The listing builds one solid part. Answer for the finished solid, in the listing's coordinates (mm). Face numbers are marked on the shaded views. Coordinates: 2 decimals unless noted, no trailing zeros. Order: outer loops, then holes, each group sorted by start corner. A loop starts at its lowest first (then second) coordinate and runs counter-clockwise, first axis right, second up. Notation, with made-up numbers: (65, -3.5) -> (100, -3.5) arc R17 cw to (100, 16.5) -> close; hole circle Ø3 at (-5.5, 78.5). An arc over 180 degrees is marked (long way). Answer in a Markdown table with one row per item.
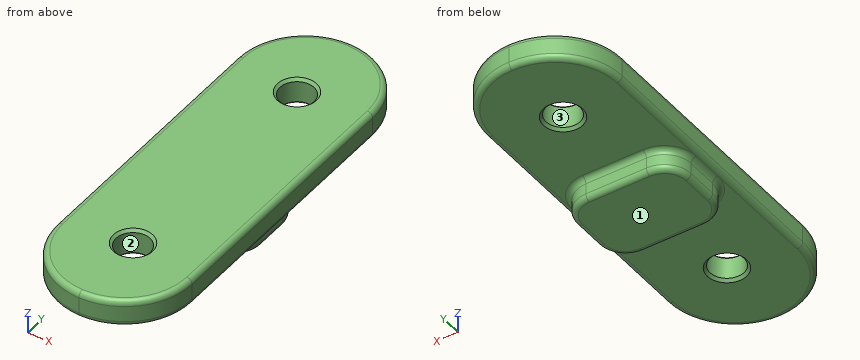
```python
from build123d import *

# Parameters (mm, degrees)
SKETCH1_W        = 25.4
SKETCH1_H        = 75.4
SKETCH1_R        = 3.2
MAINBODY_DEPTH   = 5
SKETCH2_W        = 21.4
SKETCH2_H        = 16
RIBSUPPORT_DEPTH = 4
FILLET_12_7_R    = 12.7
FILLET_5_0_R     = 5
CHAMFER_0_5_SIZE = 0.5
FILLET_1_0_R     = 1


with BuildPart() as part:
    # Sketch1 → mainBody (new body)
    with BuildSketch(Plane.XY):
        with Locations((0, 22.7)):
            Rectangle(SKETCH1_W, SKETCH1_H)
        Circle(SKETCH1_R, mode=Mode.SUBTRACT)
        with Locations((0, 45.4)):
            Circle(SKETCH1_R, mode=Mode.SUBTRACT)
    extrude(amount=MAINBODY_DEPTH)

    # Sketch2 → ribSupport (add)
    with BuildSketch(Plane(origin=(0, 0, 0), x_dir=(-1, 0, 0), z_dir=(0, 0, -1))):
        with Locations((0, 22.7)):
            Rectangle(SKETCH2_W, SKETCH2_H)
    extrude(amount=RIBSUPPORT_DEPTH)

    # Fillet-12.7
    fillet_12_7_edges = [part.edges().sort_by_distance(p)[0] for p in [
        (-12.7, -15, 2.5),
        (12.7, -15, 2.5),
        (-12.7, 60.4, 2.5),
        (12.7, 60.4, 2.5),
    ]]
    fillet(fillet_12_7_edges, radius=FILLET_12_7_R - 0.0001)  # a hair under: the kernel refuses the full size

    # Fillet-5.0
    fillet_5_0_edges = [part.edges().sort_by_distance(p)[0] for p in [
        (10.7, 30.7, -2),
        (10.7, 14.7, -2),
        (-10.7, 14.7, -2),
        (-10.7, 30.7, -2),
    ]]
    fillet(fillet_5_0_edges, radius=FILLET_5_0_R)

    # Chamfer-0.5
    chamfer_0_5_edges = [part.edges().sort_by_distance(p)[0] for p in [
        (-3.2, 0, 0),
        (-3.2, 0, 5),
        (-3.2, 45.4, 0),
        (-3.2, 45.4, 5),
    ]]
    chamfer(chamfer_0_5_edges, length=CHAMFER_0_5_SIZE)

    # Fillet-1.0
    fillet_1_0_edges = [part.edges().sort_by_distance(p)[0] for p in [
        (-12.7, 22.7, 0),
        (12.7, 22.7, 0),
        (8.98028541, 56.68028541, 0),
        (-8.98028541, 56.68028541, 0),
        (8.98028541, -11.28028541, 0),
        (-8.98028541, -11.28028541, 0),
        (-12.7, 22.7, 5),
        (12.7, 22.7, 5),
        (8.98028541, 56.68028541, 5),
        (-8.98028541, 56.68028541, 5),
        (8.98028541, -11.28028541, 5),
        (-8.98028541, -11.28028541, 5),
        (0, 30.7, 0),
        (0, 30.7, -4),
        (-10.7, 22.7, 0),
        (-10.7, 22.7, -4),
        (10.7, 22.7, -4),
        (0, 14.7, -4),
        (9.235533906, 29.235533906, -4),
        (9.235533906, 16.164466094, -4),
        (-9.235533906, 16.164466094, -4),
        (-9.235533906, 29.235533906, -4),
        (0, 14.7, 0),
        (10.7, 22.7, 0),
        (-9.235533906, 29.235533906, 0),
        (-9.235533906, 16.164466094, 0),
        (9.235533906, 16.164466094, 0),
        (9.235533906, 29.235533906, 0),
    ]]
    fillet(fillet_1_0_edges, radius=FILLET_1_0_R - 0.0001)  # a hair under: the kernel refuses the full size


solid = part.part
```
(1) Flat-ended cylindrical pins translate along their axes: pin 1 (4 mm diameter, centred on x = -4.5, z = -0.5, fed in from -Y); pin 2 (2 mm diameter, centred on y = 27, z = -3, fed in from +X); pin 3 (1.5 mm diameter, centred on x = -6.5, z = 3.5, fed in from -Y). Find the tip coordinate at first contact, or state that the pin passes through.
Check values:
| item | result |
|---|---|
| pin 1 | y = -14.62 |
| pin 2 | x = 10.69 |
| pin 3 | y = -13.62 |
(2) A cutting plane is placed at B-B, the plane z = 3.25. Count the separate pieces of the cut face and the enclosed holes in it, then the cut area to 3 significant figures.
Check values:
| item | result |
|---|---|
| separate pieces | 1 |
| enclosed holes | 2 |
| area | 1,710 mm² |
(3) A cutting plane is placed at D-D, the plane z = -1.75. Determine the outline of the cut face in (x, y), then the cut area to 3 significant figures.
Check values:
| item | result |
|---|---|
| outline | (-10.7, 19.7) arc R5 ccw to (-5.7, 14.7) -> (5.7, 14.7) arc R5 ccw to (10.7, 19.7) -> (10.7, 25.7) arc R5 ccw to (5.7, 30.7) -> (-5.7, 30.7) arc R5 ccw to (-10.7, 25.7) -> close |
| area | 321 mm² |
(4) A cutting plane is placed at A-A, the plane y = 0. Determine the outline of the cut face in (x, z), then the cut area to 3 significant figures.
Check values:
| item | result |
|---|---|
| outline | (-12.7, 1) arc R1 ccw to (-11.7, 0) -> (-3.7, 0) -> (-3.2, 0.5) -> (-3.2, 4.5) -> (-3.7, 5) -> (-11.7, 5) arc R1 ccw to (-12.7, 4) -> close; (3.2, 0.5) -> (3.7, 0) -> (11.7, 0) arc R1 ccw to (12.7, 1) -> (12.7, 4) arc R1 ccw to (11.7, 5) -> (3.7, 5) -> (3.2, 4.5) -> close |
| area | 93.6 mm² |
(5) A cutting plane is placed at C-C, the plane y = 35. Determine the outline of the cut face in (x, z).
Check values:
| item | result |
|---|---|
| outline | (-12.7, 1) arc R1 ccw to (-11.7, 0) -> (11.7, 0) arc R1 ccw to (12.7, 1) -> (12.7, 4) arc R1 ccw to (11.7, 5) -> (-11.7, 5) arc R1 ccw to (-12.7, 4) -> close |
(6) Find the intervals of material crossed by line 1 along Y through (x, z) = (0, 3); line 2 along Z through (x, y) = (-3, -11); line 3 along Y through (x, z) = (1.5, -1.25), in increasing order. Write a range as from..to.
Check values:
| item | result |
|---|---|
| line 1 | -15..-3.2, 3.2..42.2, 48.6..60.4 |
| line 2 | 0..5 |
| line 3 | 14.7..30.7 |
(7) For a pull along Y with two mould halves and no side action, classify the marked faces 1, 2 and 3 as released by +Y, released by -Y, zero draft, split by the parting line, or undercut.
Check values:
| item | result |
|---|---|
| face 1 | zero draft |
| face 2 | undercut |
| face 3 | undercut |
